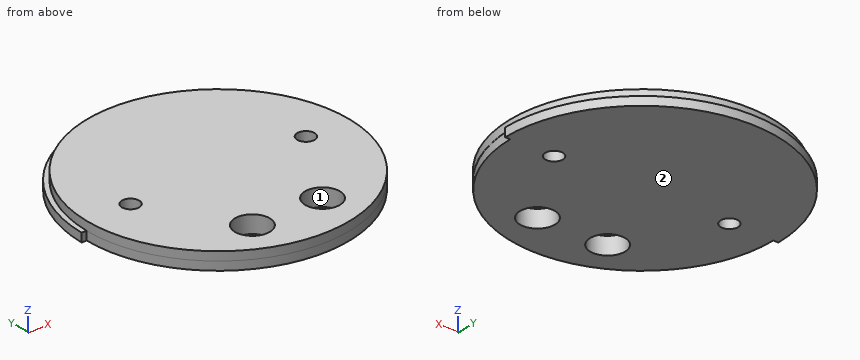
from build123d import *

# Parameters (mm, degrees)
SKETCH1_R           = 49.5046
BOSS_EXTRUDE1_DEPTH = 3.175
SKETCH2_R           = 47.6885
BOSS_EXTRUDE2_DEPTH = 3.175
SKETCH3_R           = 3.175
SKETCH3_R_2         = 6.35
CUT_EXTRUDE1_DEPTH  = 7.35
CUT_EXTRUDE2_DEPTH  = 4.175


with BuildPart() as part:
    # Sketch1 → Boss-Extrude1 (new body)
    with BuildSketch(Plane.XY):
        Circle(SKETCH1_R)
    extrude(amount=BOSS_EXTRUDE1_DEPTH)

    # Sketch2 → Boss-Extrude2 (add)
    with BuildSketch(Plane.XY.offset(3.175)):
        Circle(SKETCH2_R)
    extrude(amount=BOSS_EXTRUDE2_DEPTH)

    # Sketch3 → Cut-Extrude1 (cut, through all)
    with BuildSketch(Plane.XY.offset(6.35)):
        with Locations((-31.75, 0)):
            Circle(SKETCH3_R)
        with Locations((31.75, 0)):
            Circle(SKETCH3_R)
        with Locations((-12.7, -31.235352443)):
            Circle(SKETCH3_R_2)
        with Locations((12.7, -31.235352443)):
            Circle(SKETCH3_R_2)
    extrude(amount=-CUT_EXTRUDE1_DEPTH, mode=Mode.SUBTRACT)

    # Sketch4 → Cut-Extrude2 (cut, through all)
    with BuildSketch(Plane.XY.offset(3.175)):
        with BuildLine():
            Line((-50.165, 0), (-47.625, 0))
            ThreePointArc((-47.625, 0), (0, -47.625), (47.625, 0))
            Line((47.625, 0), (50.165, 0))
            ThreePointArc((50.165, 0), (0, -50.165), (-50.165, 0))
        make_face()
    extrude(amount=-CUT_EXTRUDE2_DEPTH, mode=Mode.SUBTRACT)


solid = part.part
For this review, take the finished solid that the model builds, in its own axes (mm). Face numbers are marked on the shaded views. Coordinates: 2 decimals unless noted, no trailing zeros. Loops run counter-clockwise (first coordinate to the right, second up) from the corner with the lowest first, then second, coordinate; pieces in that order, holes last. Notation, with made-up numbers: (68, 89) - (111, 89) arc R21 cw to (111, 106) - close; hole circle Ø5 at (25, 40.5). An arc over 180 degrees is marked (long way). Use a Markdown table: item, result. Add a question column.
Item 1: We need section C-C (z = 1.25). Give the boundary of the cut face in (x, y) (3 decimals), and give its area (3 significant figures).
Item 2: We need section A-A (y = -33). Give the boundary of the cut face in (x, z) (3 decimals).
Item 3: For line 1 (X direction, y = 0.5, z = 5); line 2 (Y direction, x = -14.5, z = 3.5); line 3 (Y direction, x = 15, z = 2.25), list the stretches that pass through material, from the lowest coordinate up.
Item 4: Mouldability with a two-part tool opening along Y and no side actions: class the marked faces 1 and 2 as pulls with the +Y half, pulls with the -Y half, needs draft (parallel to the pull), parting line crosses it, or undercut.
Item 5: We need section B-B (x = 30). Give the boundary of the cut face in (y, z) (3 decimals), and give its area (3 significant figures).
Item 6: Insertion check: pin 1 Ø1.5 at (y, z) = (-16.5, 4.5) entering from +X; pin 2 Ø3 at (y, z) = (11.5, 1.5) entering from +X; pin 3 Ø5 at (x, y) = (31.75, 0) entering from +Z; pin 4 Ø0.9 at (x, z) = (-48.5, 2) entering from -Y. Each pin has a flat end and moves straight along its axis. Give the tip position at first contact, or say it passes through.
Results list:
| question | item | result |
|---|---|---|
| 1 | outline | (-49.505, 0) - (-47.625, 0) arc R47.625 ccw to (47.625, 0) - (49.505, 0) arc R49.505 ccw to start; hole circle Ø6.35 at (-31.75, 0); hole circle Ø12.7 at (-12.7, -31.235); hole circle Ø12.7 at (12.7, -31.235); hole circle Ø6.35 at (31.75, 0) |
| 1 | area | 7,100 mm^2 |
| 2 | outline | (-34.427, 3.175) - (-34.339, 3.175) - (-34.339, 0) - (-18.8, 0) - (-18.8, 6.35) - (-34.427, 6.35) - close; (-6.6, 0) - (6.6, 0) - (6.6, 6.35) - (-6.6, 6.35) - close; (18.8, 0) - (34.339, 0) - (34.339, 3.175) - (34.427, 3.175) - (34.427, 6.35) - (18.8, 6.35) - close |
| 3 | line 1 | x = -47.69 to -34.89, -28.61 to 28.61, 34.89 to 47.69 |
| 3 | line 2 | y = -45.43 to -37.32, -25.15 to 45.43 |
| 3 | line 3 | y = -45.2 to -37.15, -25.32 to 47.18 |
| 4 | face 1 | undercut |
| 4 | face 2 | needs draft |
| 5 | outline | (-37.07, 3.175) - (-36.988, 3.175) - (-36.988, 0) - (-2.649, 0) - (-2.649, 6.35) - (-37.07, 6.35) - close; (2.649, 0) - (39.379, 0) - (39.379, 3.175) - (37.07, 3.175) - (37.07, 6.35) - (2.649, 6.35) - close |
| 5 | area | 444 mm^2 |
| 6 | pin 1 | stops at x = 45.01 |
| 6 | pin 2 | stops at x = 48.48 |
| 6 | pin 3 | passes through |
| 6 | pin 4 | stops at y = 0 |
